```python
from build123d import *

# Parameters (mm, degrees)
F0_W     = 24.1608545184
F0_H     = 14.0407383442
F0_W_2   = 28.265745379
F1_DEPTH = 1150
F2_T     = -2.5


with BuildPart() as f1:
    # F0 (on Front) → F1 (new body)
    with BuildSketch(Plane.XZ):
        Polygon((-49.6395677328, 42.5944775343), (-49.6395677328, 14.0407383442), (-25.4787132144, 14.0407383442), (27.8118383139, 14.0407383442), (56.077583693, 14.0407383442), (84.343329072, 14.0407383442), (84.343329072, 84.5464840531), (-49.6395677328, 84.5464840531), align=None)
        with Locations((-37.5591404736, 7.0203691721)):
            Rectangle(F0_W, F0_H)
        with Locations((70.2104563825, 7.0203691721)):
            Rectangle(F0_W_2, F0_H)
    extrude(amount=F1_DEPTH)

    # F2
    f2_openings = [f1.faces().sort_by_distance(p)[0] for p in [
        (17.351881, -575, 84.546484),
    ]]
    offset(amount=F2_T, openings=f2_openings, kind=Kind.INTERSECTION)


solid = f1.part
```
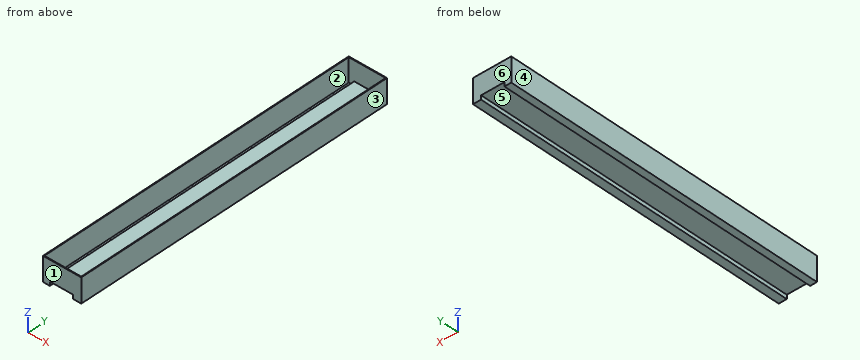
Design review of the part built by this model. Coordinates are the model's own, in mm. Face numbers are marked on the shaded views. A direction names the side the tool comes from. Round coordinates to 2 decimals unless told otherwise and drop trailing zeros. Order: outer loops, then holes, each group sorted by start corner. A loop starts at its lowest first (then second) coordinate and runs counter-clockwise, first axis right, second up. Notation, with made-up numbers: (-6.75, 30) - (38.25, 30) arc R24 ccw to (38.25, 44) - close; hole circle Ø2 at (32, -18.5). An arc over 180 degrees is marked (long way). One line per question, with ' | ' between items.
Item 1: Take a section at A-A, the plane z = 65.5. Write out the cut boundary in (x, y).
Checks:
outline: (-49.64, -1150) - (84.34, -1150) - (84.34, 0) - (-49.64, 0) - close; hole (-47.14, -1147.5) - (81.84, -1147.5) - (81.84, -2.5) - (-47.14, -2.5) - close
Item 2: Take a section at D-D, the plane x = 72. Write out the cut boundary in (y, z).
Checks:
outline: (-1150, 0) - (0, 0) - (0, 84.55) - (-2.5, 84.55) - (-2.5, 2.5) - (-1147.5, 2.5) - (-1147.5, 84.55) - (-1150, 84.55) - close
Item 3: Take a section at C-C, the plane y = -136. Write out the cut boundary in (x, z).
Checks:
outline: (-49.64, 0) - (-25.48, 0) - (-25.48, 14.04) - (56.08, 14.04) - (56.08, 0) - (84.34, 0) - (84.34, 84.55) - (81.84, 84.55) - (81.84, 2.5) - (58.58, 2.5) - (58.58, 16.54) - (-27.98, 16.54) - (-27.98, 2.5) - (-47.14, 2.5) - (-47.14, 84.55) - (-49.64, 84.55) - close
Item 4: Take a section at B-B, the plane x = 27.5. Write out the cut boundary in (y, z), then the cut area to 3 significant figures.
Checks:
outline: (-1150, 14.04) - (0, 14.04) - (0, 84.55) - (-2.5, 84.55) - (-2.5, 16.54) - (-1147.5, 16.54) - (-1147.5, 84.55) - (-1150, 84.55) - close | area: 3,220 mm²
Item 5: For P1, Ø18.5, axis at x = 71.5, y = -676, coming from the +Z side; P2, Ø24.5, axis at x = 11.5, y = -846, coming from the -Z side, all flat-tipped, find the tip position at first contact; note any pin that passes through.
Checks:
P1: z = 2.5 | P2: z = 14.04
Item 6: Wall thickness on line 1 (Y direction, x = 36.5, z = 46.5); line 2 (X direction, y = -483.5, z = 74.5); line 3 (X direction, y = -559.5, z = 10): over which ranges is each line inside the solid? List them lowest first. Write a range as [from, to].
Checks:
line 1: [-1150, -1147.5], [-2.5, 0] | line 2: [-49.64, -47.14], [81.84, 84.34] | line 3: [-49.64, -47.14], [-27.98, -25.48], [56.08, 58.58], [81.84, 84.34]
Item 7: Machinability: for the marked faces 1 and 2, which of the approach directions +Z, -Z, +X, -X, +Y, -Y give a long, thin tool a straight path to every point of the face, cutting with its end or side? Answer none if there is none.
Checks:
face 1: +Z, -Z, +X, -X, -Y | face 2: +Z
Item 8: Draft analysis for pull direction X (two halves, no side actions). For the marked faces 3, 4, 5 and 6, state which applies: +X half, -X half, draft (parallel to the pull), parting line (faces both ways), or undercut.
Checks:
face 3: +X half | face 4: -X half | face 5: undercut | face 6: draft
